Check sheet for the modelled part. Datum: model origin and axes. Units: mm. Coordinates: 2 decimals unless noted, no trailing zeros. Order: outer loops, then holes, each group sorted by start corner. A loop starts at its lowest first (then second) coordinate and runs counter-clockwise, first axis right, second up. Notation, with made-up numbers: M 88,30.5 L 94,30.5 A15 cw 94,56.5 Z; hole C 5.25,-16.75 d11. An arc over 180 degrees is marked long. Answer in a Markdown table with one row per item. Add a question column.
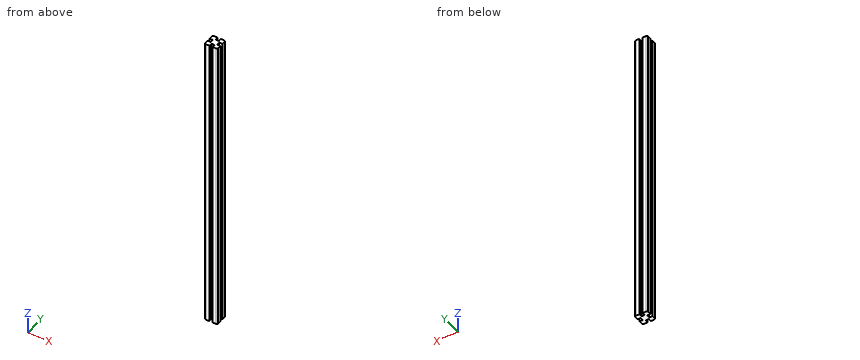
from build123d import *

# Parameters (mm, degrees)
BOSS_EXTRUDE1_DEPTH = 940


with BuildPart() as part:
    # Sketch1 → Boss-Extrude1 (new body)
    with BuildSketch(Plane.XY):
        with BuildLine():
            Line((-15.5, -20), (-5, -20))
            Line((-5, -20), (-5, -10))
            Line((-5, -10), (5, -10))
            Line((5, -10), (5, -20))
            Line((5, -20), (15.5, -20))
            ThreePointArc((15.5, -20), (18.681980515, -18.681980515), (20, -15.5))
            Line((20, -15.5), (20, -5))
            Line((20, -5), (10, -5))
            Line((10, -5), (10, 5))
            Line((10, 5), (20, 5))
            Line((20, 5), (20, 15.5))
            ThreePointArc((20, 15.5), (18.681980515, 18.681980515), (15.5, 20))
            Line((15.5, 20), (5, 20))
            Line((5, 20), (5, 10))
            Line((5, 10), (-5, 10))
            Line((-5, 10), (-5, 20))
            Line((-5, 20), (-8, 20))
            Line((-8, 20), (-15, 20))
            Line((-15, 20), (-15.5, 20))
            ThreePointArc((-15.5, 20), (-18.681980515, 18.681980515), (-20, 15.5))
            Line((-20, 15.5), (-20, 5))
            Line((-20, 5), (-10, 5))
            Line((-10, 5), (-10, -5))
            Line((-10, -5), (-20, -5))
            Line((-20, -5), (-20, -15.5))
            ThreePointArc((-20, -15.5), (-18.681980515, -18.681980515), (-15.5, -20))
        make_face()
    extrude(amount=BOSS_EXTRUDE1_DEPTH)


solid = part.part
1. Section check A-A on z = 709.5. Enter the section's corners in (x, y), then the cut area to 3 significant figures.
2. Scan lines: line 1 (Y direction, x = -16, z = 208); line 2 (Y direction, x = 1.5, z = 169.5). Record each from-to range of solid material in increasing order.
3. Go/stop test with flat-tipped pins: pin 1 Ø5 at (y, z) = (-1, 354) entering from -X; pin 2 Ø8 at (x, z) = (0.5, 356.5) entering from -Y; pin 3 Ø2 at (y, z) = (1.5, 399) entering from +X. Record where each tip stops, or that it passes through.
Result sheet:
| question | item | result |
|---|---|---|
| 1 | outline | M -20,-15.5 A4.5 ccw -15.5,-20 L -5,-20 L -5,-10 L 5,-10 L 5,-20 L 15.5,-20 A4.5 ccw 20,-15.5 L 20,-5 L 10,-5 L 10,5 L 20,5 L 20,15.5 A4.5 ccw 15.5,20 L 5,20 L 5,10 L -5,10 L -5,20 L -15.5,20 A4.5 ccw -20,15.5 L -20,5 L -10,5 L -10,-5 L -20,-5 Z |
| 1 | area | 1,180 mm^2 |
| 2 | line 1 | -19.97 to -5, 5 to 19.97 |
| 2 | line 2 | -10 to 10 |
| 3 | pin 1 | x = -10 |
| 3 | pin 2 | y = -10 |
| 3 | pin 3 | x = 10 |
